Drawing for the job (mm, zero at the part's lowest x, y, z). Round coordinates to 2 decimals unless told otherwise and drop trailing zeros. Write each loop counter-clockwise with the first axis right and the second up, starting at its lowest first coordinate (ties: lowest second). Pieces come first, ordered by that corner, then holes. Notation, with made-up numbers: (65.25, -8.75) - (98.25, -8.75) arc R17 ccw to (98.25, 4.25) - close; hole circle Ø5 at (72.5, -30). An arc over 180 degrees is marked (long way). Answer in a Markdown table with one row per item.
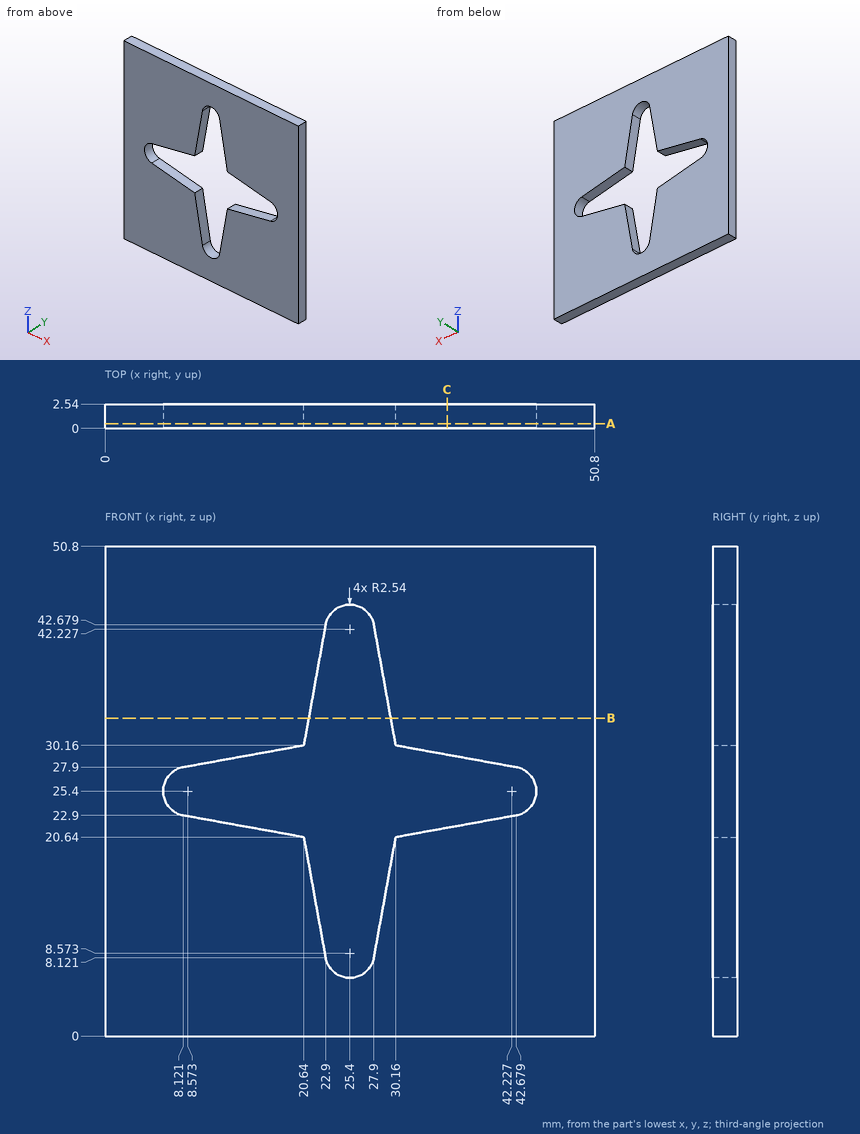
Q1. Drill centre lines: line 1 (X direction, y = 0.9, z = 19.5) (1 decimal); line 2 (Z direction, x = 43.5, y = 1.25). Where is each one in solid material? Low to high.
Computed:
| item | result |
|---|---|
| line 1 | x = 0 to 20.8, 30 to 50.8 |
| line 2 | z = 0 to 23.2, 27.6 to 50.8 |
Q2. Saw through at A-A on y = 0.5. List the corners of the cut face in (x, z).
Computed:
| item | result |
|---|---|
| outline | (0, 0) - (50.8, 0) - (50.8, 50.8) - (0, 50.8) - close; hole (8.12, 22.9) - (20.64, 20.64) - (22.9, 8.12) arc R2.54 ccw to (27.9, 8.12) - (30.16, 20.64) - (42.68, 22.9) arc R2.54 ccw to (42.68, 27.9) - (30.16, 30.16) - (27.9, 42.68) arc R2.54 ccw to (22.9, 42.68) - (20.64, 30.16) - (8.12, 27.9) arc R2.54 ccw to start |
Q3. Flat gauge pin, fed straight in: pin 1 (8 mm diameter, centred on x = 16, z = 20, fed in from -Y). Where does the tip first touch, or does it go through?
Computed:
| item | result |
|---|---|
| pin 1 | stops at y = 0 |
Q4. Saw through at C-C on x = 35.5. List the corners of the cut face in (y, z) (1 decimal), then the cut area to 3 significant figures.
Computed:
| item | result |
|---|---|
| outline | (0, 0) - (2.5, 0) - (2.5, 21.6) - (0, 21.6) - close; (0, 29.2) - (2.5, 29.2) - (2.5, 50.8) - (0, 50.8) - close |
| area | 110 mm2 |
Q5. Saw through at B-B on z = 33. List the corners of the cut face in (x, y).
Computed:
| item | result |
|---|---|
| outline | (0, 0) - (21.15, 0) - (21.15, 2.54) - (0, 2.54) - close; (29.65, 0) - (50.8, 0) - (50.8, 2.54) - (29.65, 2.54) - close |
